For this review, take the finished solid that the model builds, in its own axes (mm). A direction names the side the tool comes from. Coordinates: 2 decimals unless noted, no trailing zeros.
1. Take a section at C-C, the plane y = 3. Count the separate pieces of the cut face and the enclosed holes in it, then the cut area to 3 significant figures.
2. To check wall thickness, follow probe 1 along X at (y, z) = (0.75, -10.45); probe 2 along X at (y, z) = (3.3, -10.45) (3 decimals); probe 3 along Z at (x, y) = (-12.5, 0.7). State the ranges of each line that lie inside material, in increasing order.
3. Machinability: for faces 5 (the face through (8.352, 1.676, -5.606)), 6 (the face through (-14.62, 3.82, -12.39)), 7 (the face through (7.05, 4.46, -4.83)), which of the approach directions +Z, -Z, +X, -X, +Y, -Y give a long, thin tool a straight path to every point of the face, cutting with its end or side? Answer none if there is none.
4. Clearance check with flat-ended pins moving along their axes: P1, Ø4, axis at x = 0, z = 4.5, coming from the +Y side; P2, Ø2.5, axis at x = 12.5, z = -10.45, coming from the +Y side; P3, Ø1.7, axis at x = 12, z = 11.5, coming from the +Y side; P4, Ø4.5, axis at x = -12.5, z = -10.45, coming from the -Y side. State where each tip first meets the part, or that it passes through.
5. Mouldability with a two-part tool opening along Z and no side actions: class faces 1 (the face through (16.5, 2, 0)), 2 (the face through (-0.23, 4.99, 13.86)), 3 (the face through (14, 2.1, -9)), 4 (the face through (0, 2, -14.35)) as pulls with the +Z half, pulls with the -Z half, needs draft (parallel to the pull), parting line crosses it, or undercut.
```python
from build123d import *

# Parameters (mm, degrees)
SKETCH1_W                      = 33
SKETCH1_H                      = 28.7
BOSS_EXTRUDE1_DEPTH            = 5.5
CBORE_FOR_M3_SHCS1_D           = 3.4
CBORE_FOR_M3_SHCS1_CBORE_D     = 5.75
CBORE_FOR_M3_SHCS1_CBORE_DEPTH = 3.4
CBORE_FOR_M3_SHCS2_D           = 3.4
CBORE_FOR_M3_SHCS2_CBORE_D     = 5.75
CBORE_FOR_M3_SHCS2_CBORE_DEPTH = 3.4
SKETCH9_R                      = 11.75
SKETCH9_R_2                    = 10.25
BOSS_EXTRUDE2_DEPTH            = 2
FILLET1_R                      = 1
CHAMFER1_SIZE                  = 1


with BuildPart() as part:
    # Sketch1 → Boss-Extrude1 (new body)
    with BuildSketch(Plane(origin=(0, 0, 0), x_dir=(1, 0, 0), z_dir=(0, 1, 0))):
        Rectangle(SKETCH1_W, SKETCH1_H)
    extrude(amount=BOSS_EXTRUDE1_DEPTH)

    # CBORE for M3 SHCS1 (through all)
    with Locations(Plane(origin=(0, 5.5, 0), x_dir=(1, 0, 0), z_dir=(0, 1, 0))):
        with Locations((-12.5, 10.45), (12.5, 10.45), (12.5, -10.45), (-12.5, -10.45)):
            CounterBoreHole(CBORE_FOR_M3_SHCS1_D / 2, CBORE_FOR_M3_SHCS1_CBORE_D / 2, CBORE_FOR_M3_SHCS1_CBORE_DEPTH)

    # CBORE for M3 SHCS2 (through all)
    with Locations(Plane(origin=(0, 0, 0), x_dir=(-1, 0, 0), z_dir=(0, -1, 0))):
        with Locations((-5.480077554, -5.480077554), (5.480077554, -5.480077554), (5.480077554, 5.480077554), (-5.480077554, 5.480077554)):
            CounterBoreHole(CBORE_FOR_M3_SHCS2_D / 2, CBORE_FOR_M3_SHCS2_CBORE_D / 2, CBORE_FOR_M3_SHCS2_CBORE_DEPTH)

    # Sketch9 → Boss-Extrude2 (add)
    with BuildSketch(Plane(origin=(0, 5.5, 0), x_dir=(1, 0, 0), z_dir=(0, 1, 0))):
        with Locations(Location((0, 0, 0), (0, 0, 270))):
            Circle(SKETCH9_R)
        with Locations(Location((0, 0, 0), (0, 0, 270))):
            Circle(SKETCH9_R_2, mode=Mode.SUBTRACT)
    extrude(amount=BOSS_EXTRUDE2_DEPTH)

    # Fillet1
    fillet1_edges = [part.edges().sort_by_distance(p)[0] for p in [
        (0, 5.5, -11.75),
        (0, 7.5, -11.75),
    ]]
    fillet(fillet1_edges, radius=FILLET1_R - 0.0001)  # a hair under: the kernel refuses the full size

    # Chamfer1
    chamfer1_edges = [part.edges().sort_by_distance(p)[0] for p in [
        (16.5, 5.5, 0),
        (0, 5.5, -14.35),
        (-16.5, 5.5, 0),
        (0, 5.5, 14.35),
    ]]
    chamfer(chamfer1_edges, length=CHAMFER1_SIZE)


solid = part.part
```
Results list:
1. separate pieces: 1
1. enclosed holes: 8
1. area: 739 mm2
2. probe 1: x = -16.5 to -14.2, -10.8 to 10.8, 14.2 to 16.5
2. probe 2: x = -16.5 to -15.375, -9.625 to 9.625, 15.375 to 16.5
2. probe 3: z = -14.35 to -12.15, -8.75 to 8.75, 12.15 to 14.35
3. face 5: -Y
3. face 6: +Y
3. face 7: +Y, -Y
4. P1: stops at y = 5.5
4. P2: passes through
4. P3: stops at y = 2.1
4. P4: stops at y = 0
5. face 1: needs draft
5. face 2: pulls with the +Z half
5. face 3: undercut
5. face 4: pulls with the -Z half
